Source: CAD feature listing. Evaluate the final solid. Frame: model axes, mm. Face numbers are marked on the shaded views. A direction names the side the tool comes from. Coordinates: 2 decimals unless noted, no trailing zeros. Write each loop counter-clockwise with the first axis right and the second up, starting at its lowest first coordinate (ties: lowest second). Pieces come first, ordered by that corner, then holes. Notation, with made-up numbers: M 51.25,-13 L 88.25,-13 A31 ccw 88.25,15 Z; hole C -31,12.25 d4. An arc over 180 degrees is marked long. One line per item, written item: value. Start each with the question number.
Item 1: Cut plane B-B, the plane x = -167. Output: boundary loops of the cut face in (y, z).
Item 2: Ray query, L1, parallel to X at y = 25, z = -18; L2, parallel to Z at x = 204, y = 22; L3, parallel to X at y = 118, z = 128. Return the intervals inside material, ascending. Write a range as from..to.
Item 3: Cut plane A-A, the plane y = 149. Output: boundary loops of the cut face in (x, z).
Item 4: Cut plane C-C, the plane z = -67.5. Output: boundary loops of the cut face in (x, y).
Item 5: Mould query, pull axis Z, two halves, no side actions, for the marked faces 4, 5, 6 and 7. Classes: released by +Z, released by -Z, zero draft, split by the parting line, or undercut.
Item 6: Pin query (flat end, axial travel): P1, Ø10, axis at x = 23.5, y = 7, coming from the -Z side; P2, Ø10, axis at y = 44.5, z = -6.5, coming from the -X side; P3, Ø6, axis at y = 36.5, z = 90, coming from the +X side. Return the tip coordinate at first contact, or that it passes through.
Item 7: Cut plane D-D, the plane y = 7. Output: boundary loops of the cut face in (x, z).
Item 8: Set-up query: the marked faces 1, 2 and 3. Return all of +Z, -Z, +X, -X, +Y, -Y with unobstructed straight access to the full face (end or side cutting, diameter ignored); none if empty.
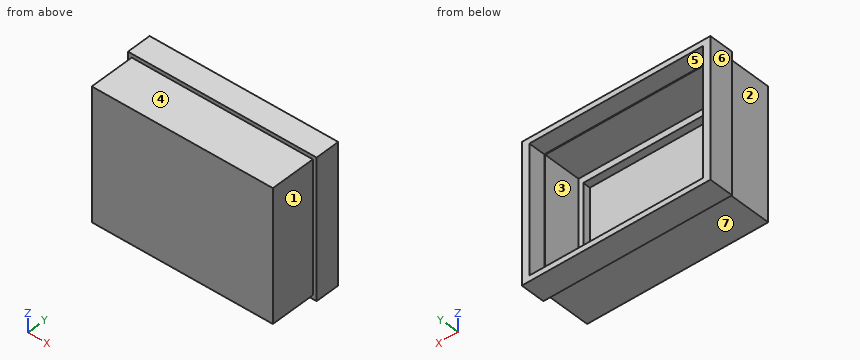
```python
from build123d import *

# Parameters (mm, degrees)
SKETCH2_W           = 500
SKETCH2_H           = 370
SKETCH2_W_2         = 430
SKETCH2_H_2         = 300
BOSS_EXTRUDE1_DEPTH = 120
SKETCH4_W           = 500
SKETCH4_H           = 370
SKETCH4_W_2         = 460
SKETCH4_H_2         = 340
BOSS_EXTRUDE2_DEPTH = 45
SKETCH5_W           = 500
SKETCH5_H           = 370
BOSS_EXTRUDE3_DEPTH = 20
SKETCH6_W           = 500
SKETCH6_H           = 370
SKETCH6_W_2         = 480
SKETCH6_H_2         = 350
CUT_EXTRUDE1_DEPTH  = 120
SKETCH8_W           = 455
SKETCH8_H           = 335
CUT_EXTRUDE2_DEPTH  = 100


with BuildPart() as part:
    # Sketch2 → Boss-Extrude1 (new body)
    with BuildSketch(Plane(origin=(0, 0, 0), x_dir=(1, 0, 0), z_dir=(0, 1, 0))):
        Rectangle(SKETCH2_W, SKETCH2_H)
        Rectangle(SKETCH2_W_2, SKETCH2_H_2, mode=Mode.SUBTRACT)
    extrude(amount=BOSS_EXTRUDE1_DEPTH)

    # Sketch4 → Boss-Extrude2 (add)
    with BuildSketch(Plane(origin=(0, 120, 0), x_dir=(1, 0, 0), z_dir=(0, 1, 0))):
        Rectangle(SKETCH4_W, SKETCH4_H)
        Rectangle(SKETCH4_W_2, SKETCH4_H_2, mode=Mode.SUBTRACT)
    extrude(amount=BOSS_EXTRUDE2_DEPTH)

    # Sketch5 → Boss-Extrude3 (add)
    with BuildSketch(Plane.XZ):
        Rectangle(SKETCH5_W, SKETCH5_H)
    extrude(amount=BOSS_EXTRUDE3_DEPTH)

    # Sketch6 → Cut-Extrude1 (cut)
    with BuildSketch(Plane.XZ.offset(20)):
        Rectangle(SKETCH6_W, SKETCH6_H)
        Rectangle(SKETCH6_W_2, SKETCH6_H_2, mode=Mode.SUBTRACT)
    extrude(amount=-CUT_EXTRUDE1_DEPTH, mode=Mode.SUBTRACT)

    # Sketch8 → Cut-Extrude2 (cut)
    with BuildSketch(Plane(origin=(0, 120, 0), x_dir=(1, 0, 0), z_dir=(0, 1, 0))):
        Rectangle(SKETCH8_W, SKETCH8_H)
    extrude(amount=-CUT_EXTRUDE2_DEPTH, mode=Mode.SUBTRACT)


solid = part.part
```
From the geometry:
1. outline: M -20,-175 L 100,-175 L 100,-185 L 165,-185 L 165,-170 L 120,-170 L 120,-167.5 L 20,-167.5 L 20,-150 L 0,-150 L 0,150 L 20,150 L 20,167.5 L 120,167.5 L 120,170 L 165,170 L 165,185 L 100,185 L 100,175 L -20,175 Z
2. L1: x = -240..-227.5, 227.5..240
2. L2: z = -175..-167.5, 167.5..175
2. L3: x = -250..-227.5, 227.5..250
3. outline: M -250,-185 L 250,-185 L 250,185 L -250,185 Z; hole M -230,-170 L 230,-170 L 230,170 L -230,170 Z
4. outline: M -250,100 L -240,100 L -240,-20 L 240,-20 L 240,100 L 250,100 L 250,165 L 230,165 L 230,120 L 227.5,120 L 227.5,20 L 215,20 L 215,0 L -215,0 L -215,20 L -227.5,20 L -227.5,120 L -230,120 L -230,165 L -250,165 Z
5. face 4: released by +Z
5. face 5: undercut
5. face 6: zero draft
5. face 7: released by -Z
6. P1: stops at z = -175
6. P2: stops at x = -240
6. P3: stops at x = 240
7. outline: M -240,-175 L 240,-175 L 240,175 L -240,175 Z; hole M -215,-150 L 215,-150 L 215,150 L -215,150 Z
8. face 1: +Z, -Z, +X, -Y
8. face 2: +Z, -Z, -X, -Y
8. face 3: +Y
